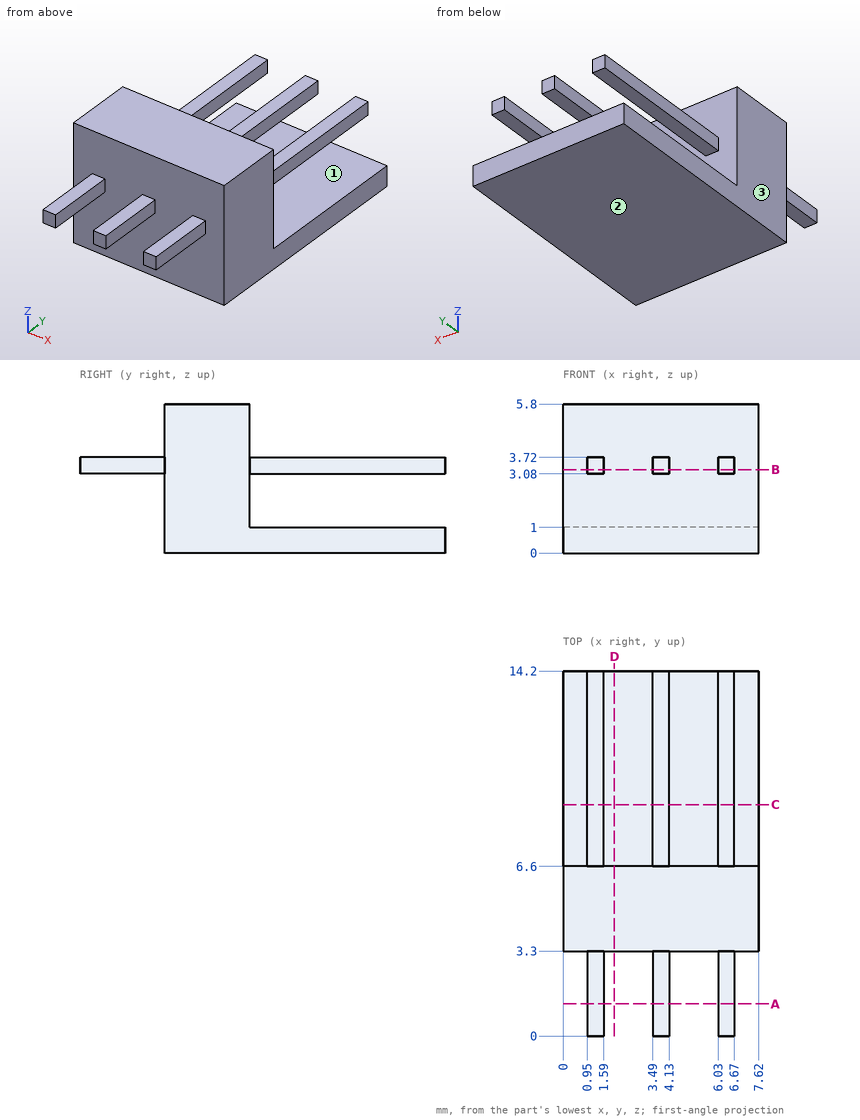
For this review, use the dimensioned drawing (mm, ordinates from the lowest corner) and the shaded views. Round coordinates to 2 decimals unless told otherwise and drop trailing zeros. Write each loop counter-clockwise with the first axis right and the second up, starting at its lowest first coordinate (ties: lowest second). Pieces come first, ordered by that corner, then holes. Notation, with made-up numbers: (59, -19.5) -> (78, -19.5) arc R6 ccw to (78, -14.5) -> close; hole circle Ø7 at (12.25, 67.25). An arc over 180 degrees is marked (long way). One line per item, written item: value. Start each with the question number.
Q1. To check wall thickness, follow probe 1 along Z at (x, y) = (1.25, 9.25); probe 2 along Y at (x, z) = (2.5, 1.55); probe 3 along Y at (x, z) = (0.5, 0.75). State the ranges of each line that lie inside material, in increasing order.
Q2. Add section B-B (z = 3.25). Give the boundary of the cut face in (x, y), then the cut area to 3 significant figures.
Q3. Add section C-C (y = 9). Give the boundary of the cut face in (x, z).
Q4. Add section D-D (x = 2). Give the boundary of the cut face in (y, z).
Q5. The part is to be moulded in two halves that separate along Z. For the marked faces 1, 2 and 3, say which applies: pulls with the +Z half, pulls with the -Z half, needs draft (parallel to the pull), parting line crosses it, or undercut.
Q6. Add section A-A (y = 1.25). Give the boundary of the cut face in (x, z).
Q7. Insertion check: P1, Ø1.5, axis at x = 3, y = 2, coming from the +Z side; P2, Ø0.7, axis at y = 1.5, z = 3.5, coming from the +X side; P3, Ø0.7, axis at y = 11, z = 3.5, coming from the -X side. Each pin has a flat end and moves straight along its axis. Give the tip position at first contact, or say it passes through.
Response:
1. probe 1: z = 0 to 1, 3.08 to 3.72
1. probe 2: y = 3.3 to 6.6
1. probe 3: y = 3.3 to 14.2
2. outline: (0, 3.3) -> (0.95, 3.3) -> (0.95, 0) -> (1.59, 0) -> (1.59, 3.3) -> (3.49, 3.3) -> (3.49, 0) -> (4.13, 0) -> (4.13, 3.3) -> (6.03, 3.3) -> (6.03, 0) -> (6.67, 0) -> (6.67, 3.3) -> (7.62, 3.3) -> (7.62, 6.6) -> (6.67, 6.6) -> (6.67, 14.2) -> (6.03, 14.2) -> (6.03, 6.6) -> (4.13, 6.6) -> (4.13, 14.2) -> (3.49, 14.2) -> (3.49, 6.6) -> (1.59, 6.6) -> (1.59, 14.2) -> (0.95, 14.2) -> (0.95, 6.6) -> (0, 6.6) -> close
2. area: 46.1 mm^2
3. outline: (0, 0) -> (7.62, 0) -> (7.62, 1) -> (0, 1) -> close; (0.95, 3.08) -> (1.59, 3.08) -> (1.59, 3.72) -> (0.95, 3.72) -> close; (3.49, 3.08) -> (4.13, 3.08) -> (4.13, 3.72) -> (3.49, 3.72) -> close; (6.03, 3.08) -> (6.67, 3.08) -> (6.67, 3.72) -> (6.03, 3.72) -> close
4. outline: (3.3, 0) -> (14.2, 0) -> (14.2, 1) -> (6.6, 1) -> (6.6, 5.8) -> (3.3, 5.8) -> close
5. face 1: undercut
5. face 2: pulls with the -Z half
5. face 3: needs draft
6. outline: (0.95, 3.08) -> (1.59, 3.08) -> (1.59, 3.72) -> (0.95, 3.72) -> close; (3.49, 3.08) -> (4.13, 3.08) -> (4.13, 3.72) -> (3.49, 3.72) -> close; (6.03, 3.08) -> (6.67, 3.08) -> (6.67, 3.72) -> (6.03, 3.72) -> close
7. P1: stops at z = 3.72
7. P2: stops at x = 6.67
7. P3: stops at x = 0.95
